```python
from build123d import *

# Parameters (mm, degrees)
BOSS_EXTRUDE1_DEPTH            = 9.525
F_5_2_5_2_DIAMETER_HOLE1_D     = 5.2
F_4_2_4_2_DIAMETER_HOLE1_D     = 4.2
F_2_5_2_5_DIAMETER_HOLE1_D     = 2.5
F_2_5_2_5_DIAMETER_HOLE1_DEPTH = 7.667982396


with BuildPart() as part:
    # Sketch1 → Boss-Extrude1 (new body)
    with BuildSketch(Plane(origin=(0, 0, 0.0762), x_dir=(-1, 0, 0), z_dir=(0, 0, -1))):
        with BuildLine():
            Line((-9.412617214, 46.18458545), (0.587382786, 46.18458545))
            ThreePointArc((0.587382786, 46.18458545), (2.110476578, 47.353297027), (1.375792677, 49.126977103))
            Line((1.375792677, 49.126977103), (-5.351179793, 51.776567317))
            ThreePointArc((-5.351179793, 51.776567317), (-18.213654114, 53.790284286), (-30.709315287, 50.135595029))
            ThreePointArc((-30.709315287, 50.135595029), (-34.537024445, 47.94381083), (-38.300389687, 45.643298402))
            ThreePointArc((-38.300389687, 45.643298402), (-39.429298758, 45.158647975), (-40.652811507, 45.047570171))
            ThreePointArc((-40.652811507, 45.047570171), (-44.686309378, 42.085440442), (-44.132804376, 37.111815022))
            ThreePointArc((-44.132804376, 37.111815022), (-43.716518775, 36.654265458), (-43.215241162, 36.291820896))
            ThreePointArc((-43.215241162, 36.291820896), (-42.428281445, 35.560296453), (-42.040186752, 34.558390211))
            ThreePointArc((-42.040186752, 34.558390211), (-41.957032136, 33.760744193), (-41.937117029, 32.959022765))
            ThreePointArc((-41.937117029, 32.959022765), (-41.88143503, 31.193095612), (-41.60760357, 29.447639934))
            ThreePointArc((-41.60760357, 29.447639934), (-41.541656296, 28.62951348), (-41.699906943, 27.824133651))
            ThreePointArc((-41.699906943, 27.824133651), (-33.057909903, 20.65839923), (-34.807142386, 31.747675507))
            ThreePointArc((-34.807142386, 31.747675507), (-37.051659352, 33.760582292), (-36.413760604, 36.707230442))
            ThreePointArc((-36.413760604, 36.707230442), (-35.419836056, 38.33724075), (-35.109301279, 40.220957226))
            ThreePointArc((-35.109301279, 40.220957226), (-34.933115189, 41.323470745), (-34.365977773, 42.285204986))
            ThreePointArc((-34.365977773, 42.285204986), (-24.606791119, 48.588208914), (-12.991191822, 48.806006202))
            ThreePointArc((-12.991191822, 48.806006202), (-11.85169268, 48.221904682), (-11.059558102, 47.215845196))
            ThreePointArc((-11.059558102, 47.215845196), (-10.384202381, 46.46367337), (-9.412617214, 46.18458545))
        make_face()
    extrude(amount=-BOSS_EXTRUDE1_DEPTH)

    # Ø5.2 (5.2) Diameter Hole1 (through all)
    with Locations(Plane.XY.offset(9.6012)):
        with Locations((40.107240677, 40.077424049)):
            Hole(F_5_2_5_2_DIAMETER_HOLE1_D / 2)

    # Ø4.2 (4.2) Diameter Hole1 (through all)
    with Locations(Plane.XY.offset(9.6012)):
        with Locations((36.026082039, 25.872797966)):
            Hole(F_4_2_4_2_DIAMETER_HOLE1_D / 2)

    # Ø2.5 (2.5) Diameter Hole1
    with Locations(Plane(origin=(0, 46.18458545, 0), x_dir=(-1, 0, 0), z_dir=(0, -1, 0))):
        with Locations((-4.401993155, -4.8387)):
            Hole(F_2_5_2_5_DIAMETER_HOLE1_D / 2, depth=F_2_5_2_5_DIAMETER_HOLE1_DEPTH)


solid = part.part
```
For this review, take the finished solid that the model builds, in its own axes (mm). A direction names the side the tool comes from. Round coordinates to 2 decimals unless told otherwise and drop trailing zeros. Order: outer loops, then holes, each group sorted by start corner. A loop starts at its lowest first (then second) coordinate and runs counter-clockwise, first axis right, second up. Notation, with made-up numbers: (58.25, 9) -> (79.25, 9) arc R3 ccw to (79.25, 14) -> close; hole circle Ø11 at (55, 6.25). An arc over 180 degrees is marked (long way). Use a Markdown table: item, result.
Item 1: Take a section at C-C (y = 27). State the section outline as (x, z) points.
Resolved:
| item | result |
|---|---|
| outline | (30.13, 0.08) -> (34.25, 0.08) -> (34.25, 9.6) -> (30.13, 9.6) -> close; (37.8, 0.08) -> (41.92, 0.08) -> (41.92, 9.6) -> (37.8, 9.6) -> close |
Item 2: Draft analysis for pull direction X (two halves, no side actions). For faces 5 (the cylindrical face through (24.76, 48.54, 4.77)), 6 (the flat face through (32, 46, 9.601)), 7 (the cylindrical face through (41.884, 31.218, 4.772)), 8 (the cylindrical face through (11.866, 48.233, 4.772)), state which applies: +X half, -X half, draft (parallel to the pull), parting line (faces both ways), or undercut.
Resolved:
| item | result |
|---|---|
| face 5 | undercut |
| face 6 | draft |
| face 7 | +X half |
| face 8 | undercut |
Item 3: Take a section at D-D (x = 14). State the section outline as (y, z) points.
Resolved:
| item | result |
|---|---|
| outline | (49.05, 0.08) -> (53.76, 0.08) -> (53.76, 9.6) -> (49.05, 9.6) -> close |
Item 4: For pin 1 (3 mm diameter, centred on y = 45.5, z = 4.5, fed in from -X); pin 2 (3 mm diameter, centred on y = 44.5, z = 2.5, fed in from +X); pin 3 (5 mm diameter, centred on y = 40.5, z = 7, fed in from -X); pin 4 (1.5 mm diameter, centred on x = 4.4, z = 4.84, fed in from +Y), all flat-tipped, find the tip position at first contact; note any pin that passes through.
Resolved:
| item | result |
|---|---|
| pin 1 | stops at x = -1.97 |
| pin 2 | stops at x = 44.16 |
| pin 3 | stops at x = 33.71 |
| pin 4 | passes through |
Item 5: Take a section at B-B (z = 7.5). State the section outline as (x, y) points, plus the area to 3 significant figures.
Resolved:
| item | result |
|---|---|
| outline | (-1.38, 49.13) arc R1.58 ccw to (-0.59, 46.18) -> (9.41, 46.18) arc R1.83 ccw to (11.06, 47.22) arc R3 cw to (12.99, 48.81) arc R21.21 cw to (34.37, 42.29) arc R3 cw to (35.11, 40.22) arc R5 ccw to (36.41, 36.71) arc R3 cw to (34.81, 31.75) arc R6 ccw (long way) to (41.7, 27.82) arc R3 cw to (41.61, 29.45) arc R14.25 ccw to (41.94, 32.96) arc R10.15 cw to (42.04, 34.56) arc R2.4 cw to (43.22, 36.29) arc R3 ccw to (44.13, 37.11) arc R5 ccw to (40.65, 45.05) arc R3.92 cw to (38.3, 45.64) arc R153.99 ccw to (30.71, 50.14) arc R29.84 ccw to (5.35, 51.78) -> close; hole circle Ø4.2 at (36.03, 25.87); hole circle Ø5.2 at (40.11, 40.08) |
| area | 368 mm² |
Item 6: Machinability: for faces 1 (the flat face through (3, 46.185, 4)), 2 (the cylindrical face through (10.396, 46.471, 4.772)), 3 (the cylindrical face through (41.958, 33.772, 4.772)), 4 (the cylindrical face through (34.94, 41.31, 4.77)), which of the approach directions +Z, -Z, +X, -X, +Y, -Y give a long, thin tool a straight path to every point of the face, cutting with its end or side? Answer none if there is none.
Resolved:
| item | result |
|---|---|
| face 1 | +Z, -Z, -X, -Y |
| face 2 | +Z, -Z, -Y |
| face 3 | +Z, -Z, +X |
| face 4 | +Z, -Z, -X |
Item 7: Take a section at A-A (y = 38). State the section outline as (x, z) points.
Resolved:
| item | result |
|---|---|
| outline | (35.56, 0.08) -> (38.54, 0.08) -> (38.54, 9.6) -> (35.56, 9.6) -> close; (41.67, 0.08) -> (44.66, 0.08) -> (44.66, 9.6) -> (41.67, 9.6) -> close |
Item 8: For line 1 along Y through (x, z) = (34.5, 7.5); line 2 along Y through (x, z) = (40.5, 3.75); line 3 along X through (y, z) = (24, 1.5), list the stretches that pass through material, from the lowest coordinate up. Write a range as [from, to].
Resolved:
| item | result |
|---|---|
| line 1 | y = [20.07, 24.43], [27.32, 31.68], [42.12, 47.97] |
| line 2 | y = [21.87, 37.51], [42.65, 45.04] |
| line 3 | x = [30.33, 35.08], [36.98, 41.73] |
